Read the model definition and answer for the solid it produces. Units are mm, in the model's axes. A direction names the side the tool comes from. Coordinates: 2 decimals unless noted, no trailing zeros. Loops run counter-clockwise (first coordinate to the right, second up) from the corner with the lowest first, then second, coordinate; pieces in that order, holes last.
from build123d import *

# Parameters (mm, degrees)
F0_R      = 35
F0_R_2    = 31.5
F1_DEPTH  = 3.5
F2_W      = 20
F2_H      = 3
F3_DEPTH  = 3.5
F4_DEPTH  = 12.5
F9_W      = 10.4753747582
F9_H      = 9.4332345761
F10_ANGLE = 280


# Not quite as in the source:
# - a feature names something its author has since deleted; it is built from what else it names


with BuildPart() as f1:
    # F0 (on Top) → F1 (new body, symmetric)
    with BuildSketch(Plane.XY):
        Circle(F0_R)
        Circle(F0_R_2, mode=Mode.SUBTRACT)
    extrude(amount=F1_DEPTH, both=True)

    # F2 (on Top) → F3 (join, symmetric)
    with BuildSketch(Plane.XY):
        with BuildLine():
            ThreePointArc((12, 38), (11.7071067812, 38.7071067812), (11, 39))
            Line((11, 39), (-11, 39))
            ThreePointArc((-11, 39), (-11.7071067812, 38.7071067812), (-12, 38))
            Line((-12, 38), (-12, 31.5))
            Line((-12, 31.5), (12, 31.5))
            Line((12, 31.5), (12, 38))
        make_face()
        with Locations((0, 35.5)):
            Rectangle(F2_W, F2_H, mode=Mode.SUBTRACT)
    extrude(amount=F3_DEPTH, both=True)

    # F2 (on Top) → F4 (cut, symmetric)
    with BuildSketch(Plane.XY):
        with Locations((0, 35.5)):
            Rectangle(F2_W, F2_H)
    extrude(amount=F4_DEPTH, both=True, mode=Mode.SUBTRACT)

    # F9 (on face) → F10 (revolve, cut)
    with BuildSketch(Plane(origin=(0, 0, 0), x_dir=(0.6427876097, 0.7660444431, 0), z_dir=(0.7660444431, -0.6427876097, 0))):
        with Locations((33.1802591681, -0.398933189)):
            Rectangle(F9_W, F9_H)
    revolve(axis=Axis((0, 0, 0), (0, 0, -1)), revolution_arc=F10_ANGLE, mode=Mode.SUBTRACT)

    # F5 (on Top) → F11 (revolve, cut)
    with BuildSketch(Plane.XY):
        Polygon((16.5, 28.5788383249), (17.8856406461, 27.7788383249), (19.0980762114, 27.0788383249), (20.7630293139, 29.9626216907), (18.1649531025, 31.4626216907), align=None)
        Polygon((16.0922047839, 24.6725162916), (17.8856406461, 27.7788383249), (16.5, 28.5788383249), (14.7065641379, 25.4725162916), align=None)
    revolve(axis=Axis((15.0315794057, 26.0354592487, 0), (0.5, 0.8660254038, 0)), mode=Mode.SUBTRACT)

    # F6 (on Top) → F12 (revolve, cut)
    with BuildSketch(Plane.XY):
        Polygon((-19.0980762114, 27.0788383249), (-17.8856406461, 27.7788383249), (-16.5, 28.5788383249), (-17.8281544713, 30.8792693496), (-20.4262306827, 29.3792693496), align=None)
        Polygon((-16.5, 28.5788383249), (-17.8856406461, 27.7788383249), (-16.1036535179, 24.6923460805), (-14.7180128719, 25.4923460805), align=None)
    revolve(axis=Axis((-13.6687379183, 23.6749485498, 0), (-0.5, 0.8660254038, 0)), mode=Mode.SUBTRACT)


solid = f1.part
Item 1: Which of the six approach directions +Z, -Z, +X, -X, +Y, -Y give full straight-line access (tool end or side, diameter ignored) to faces 4 (the face through (-10, 35, 0)), 5 (the face through (0, 39, 0)), 6 (the face through (12, 35, 0)), 7 (the face through (-17.62, 27.93, -1.29)), 8 (the face through (-12, 35, 0))?
Numbers:
face 4: +Z, -Z
face 5: +Z, -Z, +X, -X, +Y
face 6: +Z, -Z, +X, +Y
face 7: none
face 8: +Z, -Z, -X, +Y
Item 2: Find the intervals of material crossed by line 1 along X through (y, z) = (35.5, -1); line 2 along Y through (x, z) = (0, 0.75); line 3 along X through (y, z) = (33.5, -2.25), in increasing order.
Numbers:
line 1: x = -12 to -10, 10 to 12
line 2: y = 31.5 to 34, 37 to 39
line 3: x = -12 to 12
Item 3: A cutting plane is placed at D-D on z = -2.25. Determine the outline of the cut face in (x, y).
Numbers:
outline: (-22.5, 26.81) - (-20.25, 24.13) arc R31.5 cw to (20.25, 24.13) - (22.5, 26.81) arc R35 ccw to (19.19, 29.27) - (18.22, 27.59) - (14.78, 29.57) - (15.75, 31.25) arc R35 ccw to (12, 32.88) - (12, 38) arc R1 ccw to (11, 39) - (-11, 39) arc R1 ccw to (-12, 38) - (-12, 32.88) arc R35 ccw to (-15.75, 31.25) - (-14.78, 29.57) - (-18.22, 27.59) - (-19.19, 29.27) arc R35 ccw to start; hole (-10, 34) - (10, 34) - (10, 37) - (-10, 37) - close
Item 4: A cutting plane is placed at A-A on y = 34.75. Determine the outline of the cut face in (x, z).
Numbers:
outline: (-12, -3.5) - (-10, -3.5) - (-10, 3.5) - (-12, 3.5) - close; (10, -3.5) - (12, -3.5) - (12, 3.5) - (10, 3.5) - close
Item 5: Given pin 1 (3.5 mm diameter, centred on y = 35, z = -1.5, fed in from +X); pin 2 (1 mm diameter, centred on x = 7, z = 0.5, fed in from -Y); pin 3 (1 mm diameter, centred on x = 14.5, y = 34.5, fed in from -Z); pin 4 (3.5 mm diameter, centred on y = 36, z = -1.5, fed in from -X), each flat-ended and moving along its own axis, determine where each tip first touches the part or whether it passes through.
Numbers:
pin 1: stops at x = 12
pin 2: stops at y = 30.59
pin 3: passes through
pin 4: stops at x = -12
Item 6: A cutting plane is placed at B-B on z = 1. Give the number of separate pieces and of enclosed holes in the cut face, then the cut area to 3 significant figures.
Numbers:
separate pieces: 3
enclosed holes: 1
area: 185 mm2
Item 7: A cutting plane is placed at C-C on x = -5.5. Determine the outline of the cut face in (y, z).
Numbers:
outline: (31.02, -3.5) - (34, -3.5) - (34, 3.5) - (31.02, 3.5) - close; (37, -3.5) - (39, -3.5) - (39, 3.5) - (37, 3.5) - close
Item 8: Determine the mould class of faces 1 (the face through (-17.44, 30.346, 3.16)), 2 (the face through (0, 37, 0)), 3 (the face through (0, 32, 3.5)) for opening direction Y: released by +Y, released by -Y, zero draft, split by the parting line, or undercut.
Numbers:
face 1: released by +Y
face 2: undercut
face 3: zero draft
